Input: part model. Units: mm. Frame: model coordinates. A direction names the side the tool comes from. Round coordinates to 2 decimals unless told otherwise and drop trailing zeros. Order: outer loops, then holes, each group sorted by start corner. A loop starts at its lowest first (then second) coordinate and runs counter-clockwise, first axis right, second up.
Item 1: Line query: L1, parallel to Z at x = 17.45, y = 0; L2, parallel to X at y = -11, z = 53; L3, parallel to Z at x = 5.5, y = 7. Output: solid intervals per line, ascending.
Item 2: First-contact query: pin 1 (3 mm diameter, centred on x = -9, y = 3, fed in from +Z); pin 2 (1.5 mm diameter, centred on y = 4.5, z = 52.5, fed in from -X). Flat tips, straight axial feed; report the tip coordinate or a pass-through.
Item 3: Cut plane A-A on z = 61. Output: boundary loops of the cut face in (x, y).
Item 4: Reachability of faces 4 (the flat face through (4, 0, 2)), 5 (the flat face through (16, 12.5, 25)) from +Z, -Z, +X, -X, +Y, -Y: full face, straight path, thin tool, end or side. Return the list, or none.
Item 5: Cut plane B-B on y = -3.75. Output: boundary loops of the cut face in (x, z).
Item 6: Mould query, pull axis Y, two halves, no side actions, for faces 1 (the flat face through (16, -12.5, 25)), 2 (the flat face through (3, 3, 0)), 3 (the cylindrical face through (-3, 0, 1)). Classes: released by +Y, released by -Y, zero draft, split by the parting line, or undercut.
```python
from build123d import *

# Parameters (mm, degrees)
F0_R     = 3
F1_DEPTH = 2
F2_W     = 4
F2_H     = 25
F3_DEPTH = 70
F4_R     = 2.75
F5_DEPTH = 31.501
F6_R     = 12.49999


# Not quite as in the source:
# - a fillet or chamfer is up to 0.001 mm smaller than in the source, because OpenCascade refuses the exact size
# - a feature names something its author has since deleted; it is built from what else it names


with BuildPart() as f1:
    # F0 (on Top) → F1 (new body)
    with BuildSketch(Plane.XY):
        with BuildLine():
            ThreePointArc((0, -12.5), (8.8388347648, -8.8388347648), (12.5, 0))
            ThreePointArc((12.5, 0), (8.8388347648, 8.8388347648), (0, 12.5))
            ThreePointArc((0, 12.5), (-12.5, 0), (0, -12.5))
        make_face()
        with BuildLine():
            ThreePointArc((1.4953181783, 9.3815789474), (7.2268777039, 6.1662175321), (9.5, 0))
            ThreePointArc((9.5, 0), (7.2268777039, -6.1662175321), (1.4953181783, -9.3815789474))
            ThreePointArc((1.4953181783, -9.3815789474), (1.4988290876, -9.4407432173), (1.5, -9.5))
            ThreePointArc((1.5, -9.5), (-0.0592567827, -10.9988290876), (-1.4953181783, -9.3815789474))
            ThreePointArc((-1.4953181783, -9.3815789474), (-7.2268777039, -6.1662175321), (-9.5, 0))
            ThreePointArc((-9.5, 0), (-7.2268777039, 6.1662175321), (-1.4953181783, 9.3815789474))
            ThreePointArc((-1.4953181783, 9.3815789474), (-0.0592567827, 10.9988290876), (1.5, 9.5))
            ThreePointArc((1.5, 9.5), (1.4988290876, 9.4407432173), (1.4953181783, 9.3815789474))
        make_face(mode=Mode.SUBTRACT)
        with BuildLine():
            ThreePointArc((0, 12.5), (8.8388347648, 8.8388347648), (12.5, 0))
            ThreePointArc((12.5, 0), (8.8388347648, -8.8388347648), (0, -12.5))
            Line((0, -12.5), (19, -12.5))
            Line((19, -12.5), (19, 12.5))
            Line((19, 12.5), (0, 12.5))
        make_face()
        with BuildLine():
            ThreePointArc((7.859375, -1.4933936552), (6.5, 0), (7.859375, 1.4933936552))
            ThreePointArc((7.859375, 1.4933936552), (5.1016100823, 6.1622702446), (1.34e-08, 8))
            ThreePointArc((1.34e-08, 8), (-5.101610072, 6.1622702532), (-7.859375, 1.4933936552))
            ThreePointArc((-7.859375, 1.4933936552), (-6.8907350407, 1.0097184013), (-6.5, 0))
            ThreePointArc((-6.5, 0), (-6.8907350407, -1.0097184013), (-7.859375, -1.4933936552))
            ThreePointArc((-7.859375, -1.4933936552), (-5.1016100771, -6.1622702489), (0, -8))
            ThreePointArc((0, -8), (5.1016100771, -6.1622702489), (7.859375, -1.4933936552))
        make_face()
        Circle(F0_R, mode=Mode.SUBTRACT)
        with BuildLine():
            ThreePointArc((7.859375, 1.4933936552), (9.0097184013, 1.1092649593), (9.5, 0))
            ThreePointArc((9.5, 0), (7.2268777039, 6.1662175321), (1.4953181783, 9.3815789474))
            ThreePointArc((1.4953181783, 9.3815789474), (1.0179313437, 8.3982669201), (1.34e-08, 8))
            ThreePointArc((1.34e-08, 8), (5.1016100823, 6.1622702446), (7.859375, 1.4933936552))
        make_face()
        with BuildLine():
            ThreePointArc((1.4953181783, -9.3815789474), (7.2268777039, -6.1662175321), (9.5, 0))
            ThreePointArc((9.5, 0), (9.0097184013, -1.1092649593), (7.859375, -1.4933936552))
            ThreePointArc((7.859375, -1.4933936552), (5.1016100771, -6.1622702489), (0, -8))
            ThreePointArc((0, -8), (1.0179313388, -8.3982669155), (1.4953181783, -9.3815789474))
        make_face()
        with BuildLine():
            ThreePointArc((1.34e-08, 8), (-1.0179313339, 8.3982669109), (-1.4953181783, 9.3815789474))
            ThreePointArc((-1.4953181783, 9.3815789474), (-7.2268777039, 6.1662175321), (-9.5, 0))
            ThreePointArc((-9.5, 0), (-9.0097184013, 1.1092649593), (-7.859375, 1.4933936552))
            ThreePointArc((-7.859375, 1.4933936552), (-5.101610072, 6.1622702532), (1.34e-08, 8))
        make_face()
        with BuildLine():
            ThreePointArc((-9.5, 0), (-7.2268777039, -6.1662175321), (-1.4953181783, -9.3815789474))
            ThreePointArc((-1.4953181783, -9.3815789474), (-1.0179313388, -8.3982669155), (0, -8))
            ThreePointArc((0, -8), (-5.1016100771, -6.1622702489), (-7.859375, -1.4933936552))
            ThreePointArc((-7.859375, -1.4933936552), (-9.0097184013, -1.1092649593), (-9.5, 0))
        make_face()
    extrude(amount=F1_DEPTH)

    # F2 (on face) → F3 (join)
    with BuildSketch(Plane.XY.offset(2)):
        with Locations((17, 0)):
            Rectangle(F2_W, F2_H)
    extrude(amount=F3_DEPTH)

    # F4 (on face) → F5 (cut, through all)
    with BuildSketch(Plane.YZ.offset(19)):
        with Locations((0, 59.5)):
            Circle(F4_R)
    extrude(amount=-F5_DEPTH, mode=Mode.SUBTRACT)

    # F6 (radius 12.5 in the source; OpenCascade refuses exactly that, so slightly less here)
    f6_edges = [f1.edges().sort_by_distance(p)[0] for p in [
        (17, -12.5, 72),
        (17, 12.5, 72),
    ]]
    fillet(f6_edges, radius=F6_R)


solid = f1.part
```
From the geometry:
1. L1: z = 0 to 56.75, 62.25 to 72
1. L2: x = 15 to 19
1. L3: z = 0 to 2
2. pin 1: stops at z = 2
2. pin 2: stops at x = 15
3. outline: (15, -12.41) - (19, -12.41) - (19, -2.3) - (15, -2.3) - close; (15, 2.3) - (19, 2.3) - (19, 12.41) - (15, 12.41) - close
4. face 4: +Z, -X, +Y, -Y
4. face 5: +Z, -Z, +X, -X, +Y
5. outline: (-11.92, 0) - (19, 0) - (19, 71.42) - (15, 71.42) - (15, 2) - (-11.92, 2) - close
6. face 1: released by -Y
6. face 2: zero draft
6. face 3: undercut
